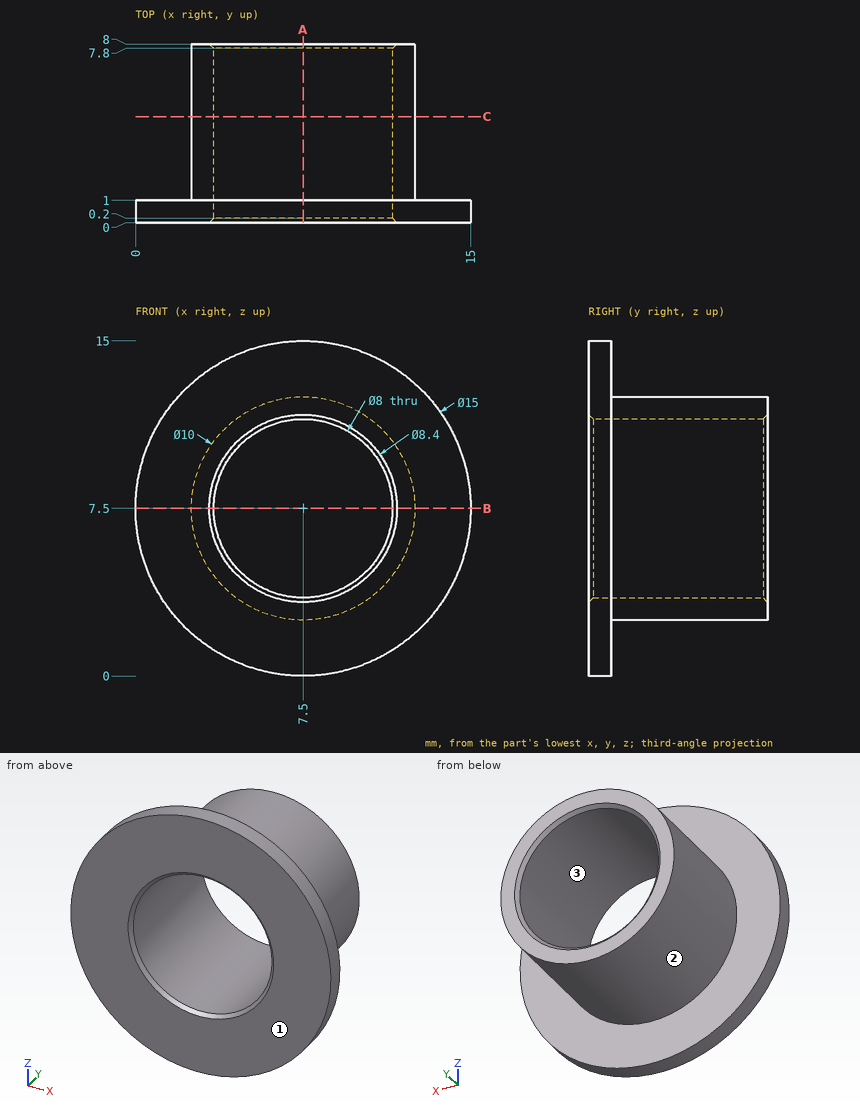
Here's the drawing with two shaded views (mm, measured from the low corner). I have some questions. Coordinates: 2 decimals unless noted, no trailing zeros. Loops run counter-clockwise (first coordinate to the right, second up) from the corner with the lowest first, then second, coordinate; pieces in that order, holes last. Notation, with made-up numbers: (6.25, 11.25) -> (12.25, 11.25) arc R4 cw to (12.25, 18.25) -> close; hole circle Ø7 at (46.5, -25). An arc over 180 degrees is marked (long way). Put each result on its own line as item: value. Start each with the question number.
Q1. If I drill on line 1 (X direction, y = 2, z = 7.5); line 2 (Y direction, x = 8.5, z = 14.25); line 3 (Z direction, x = 9.5, y = 7.25), over which ranges is the centre line in solid material (lowest first)? Write a range as [from, to].
Q2. I want a section at C-C (y = 4.75). Write out the boundary of the cut face in (x, z).
Q3. I want a section at B-B (z = 7.5). Write out the boundary of the cut face in (x, y).
Q4. Thinking about a two-plate mould opening in Z: for the marked faces 1, 2 and 3, which applies, pulls with the +Z half, pulls with the -Z half, needs draft (parallel to the pull), parting line crosses it, or undercut?
Q5. I want a section at A-A (x = 7.5). Write out the boundary of the cut face in (y, z), plus the area to 3 significant figures.
Q6. I'm going to push a flat-ended pin straight in: P1, Ø3, axis at x = 2.5, y = 4, coming from the -Z side. Where does the tip first touch, or does it pass through?
Taken from the geometry:
1. line 1: x = [2.5, 3.5], [11.5, 12.5]
1. line 2: y = [0, 1]
1. line 3: z = [2.92, 4.04], [10.96, 12.08]
2. outline: circle Ø10 at (7.5, 7.5); hole circle Ø8 at (7.5, 7.5)
3. outline: (0, 0) -> (3.3, 0) -> (3.5, 0.2) -> (3.5, 7.8) -> (3.3, 8) -> (2.5, 8) -> (2.5, 1) -> (0, 1) -> close; (11.5, 0.2) -> (11.7, 0) -> (15, 0) -> (15, 1) -> (12.5, 1) -> (12.5, 8) -> (11.7, 8) -> (11.5, 7.8) -> close
4. face 1: needs draft
4. face 2: parting line crosses it
4. face 3: undercut
5. outline: (0, 0) -> (1, 0) -> (1, 2.5) -> (8, 2.5) -> (8, 3.3) -> (7.8, 3.5) -> (0.2, 3.5) -> (0, 3.3) -> close; (0, 11.7) -> (0.2, 11.5) -> (7.8, 11.5) -> (8, 11.7) -> (8, 12.5) -> (1, 12.5) -> (1, 15) -> (0, 15) -> close
5. area: 20.9 mm2
6. P1: stops at z = 3.93
